For this review, take the finished solid that the model builds, in its own axes (mm). A direction names the side the tool comes from. Give positions to 0.01 mm unless a question says otherwise; leave off trailing zeros. Order: outer loops, then holes, each group sorted by start corner. A loop starts at its lowest first (then second) coordinate and runs counter-clockwise, first axis right, second up.
Autodesk Inventor part; units mm, degrees
ref_plane "Work Plane1" through (0, 0, -5) normal (0, 0, 1) x (1, 0, 0)
ref_plane "Work Plane2" through (0, 0, -35) normal (0, 0, -1) x (-1, 0, 0)
ref_plane "YZ Plane" through (0, 0, 0) normal (1, 0, 0) x (0, 1, 0)
sketch "Sketch1" plane through (0, 0, 0) normal (0, 0, 1) x (1, 0, 0)
  line L0 (0, 0) -> (-12, 0)
  line L1 (-12, 0) -> (-12, 1)
  line L2 (-12, 1) -> (-2.2361, 1)
  arc A0 (0, 0) -> (-2.2361, 1) centre (0, 3) ccw
  circle A1 centre (0, 3) radius 2
  dimension "d1" = 1
  dimension "d2" = 6
  dimension "d3" = 4
  dimension "d4" = 12
extrude "Extrusion1" add sketch "Sketch1" against normal blind 40
ref_plane "Work Plane1" through (0, 0, -5) normal (0, 0, 1) x (1, 0, 0)
sketch "Sketch3" plane through (0, 0, -5) normal (0, 0, 1) x (1, 0, 0)
  arc A0 (0, 0) -> (-2.2361, 1) centre (0, 3) ccw
  arc A1 (0, 0) -> (-2.2361, 1) centre (0, 3) ccw
  line L0 (-2.2361, 1) -> (-2.2361, 0)
  line L1 (-2.2361, 0) -> (0, 0)
  circle A2 centre (0, 3) radius 2
  circle A3 centre (0, 3) radius 2
  point P0 (-2.2361, 1)
extrude "Extrusion2" cut sketch "Sketch3" against normal blind 10
ref_plane "Work Plane2" through (0, 0, -35) normal (0, 0, -1) x (-1, 0, 0)
sketch "Sketch4" plane through (0, 0, -35) normal (0, 0, -1) x (-1, 0, 0)
  arc A0 (2.2361, 1) -> (0, 0) centre (0, 3) ccw
  arc A1 (2.2361, 1) -> (0, 0) centre (0, 3) ccw
  circle A2 centre (0, 3) radius 2
  circle A3 centre (0, 3) radius 2
  line L0 (2.2361, 1) -> (2.2361, 0)
  line L1 (2.2361, 0) -> (0, 0)
  point P0 (2.2361, 1)
extrude "Extrusion3" cut sketch "Sketch4" against normal blind 10
properties part number "Poker hinge 1"
1) We need section C-C on x = -8. Give the boundary of the cut face in (y, z), then the cut area to 3 significant figures.
Answer sheet:
outline: (0, -40) - (1, -40) - (1, 0) - (0, 0) - close
area: 40.0 mm2
2) Draft analysis for pull direction Z (two halves, no side actions). For faces 1 (the face through (-2, 2, -40)), 2 (the face through (0, 1, -20)), 3 (the face through (1, 1, -5)), state which applies: +Z half, -Z half, draft (parallel to the pull), parting line (faces both ways), or undercut.
Answer sheet:
face 1: -Z half
face 2: draft
face 3: undercut
3) To check wall thickness, follow line 1 (Z direction, x = 2, y = 2); line 2 (Y direction, x = 0, z = -38.3); line 3 (X direction, y = 3, z = -38.4). State the ranges of each line that lie inside material, in increasing order.
Answer sheet:
line 1: z = -40 to -35, -25 to -15, -5 to 0
line 2: y = 0 to 1, 5 to 6
line 3: x = -3 to -2, 2 to 3
4) We need section A-A on y = 3. Give the boundary of the cut face in (x, z).
Answer sheet:
outline: (-3, -40) - (-2, -40) - (-2, -35) - (-3, -35) - close; (-3, -25) - (-2, -25) - (-2, -15) - (-3, -15) - close; (-3, -5) - (-2, -5) - (-2, 0) - (-3, 0) - close; (2, -40) - (3, -40) - (3, -35) - (2, -35) - close; (2, -25) - (3, -25) - (3, -15) - (2, -15) - close; (2, -5) - (3, -5) - (3, 0) - (2, 0) - close
5) We need section D-D on z = -33. Give the boundary of the cut face in (x, y), then the cut area to 3 significant figures.
Answer sheet:
outline: (-12, 0) - (-2.24, 0) - (-2.24, 1) - (-12, 1) - close
area: 9.76 mm2
6) We need section B-B on z = -16.5. Give the boundary of the cut face in (x, y).
Answer sheet:
outline: (-12, 0) - (0, 0) arc R3 ccw (long way) to (-2.24, 1) - (-12, 1) - close; hole circle Ø4 at (0, 3)
7) Tool access review of faces 4 (the face through (-1, 1, -25)), 5 (the face through (-2.236, 0.5, -9.9)), 6 (the face through (-2, 2, 0)): name each direction out of +Z, -Z, +X, -X, +Y, -Y from which nothing blocks a thin tool from reaching the whole face with its end or side.
Answer sheet:
face 4: +X, +Y
face 5: +X, +Y, -Y
face 6: +Z, +X, -X, +Y, -Y
8) Clearance check with flat-ended pins moving along their axes: pin 1 (1.5 mm diameter, centred on y = 4.5, z = -34.5, fed in from -X); pin 2 (1.1 mm diameter, centred on y = 0.5, z = -28.5, fed in from +X); pin 3 (4 mm diameter, centred on x = -7.5, z = -6, fed in from +Y); pin 4 (3 mm diameter, centred on x = 1, y = 4, fed in from -Z). State where each tip first meets the part, or that it passes through.
Answer sheet:
pin 1: stops at x = -2.85
pin 2: stops at x = -2.24
pin 3: stops at y = 1
pin 4: stops at z = -40
